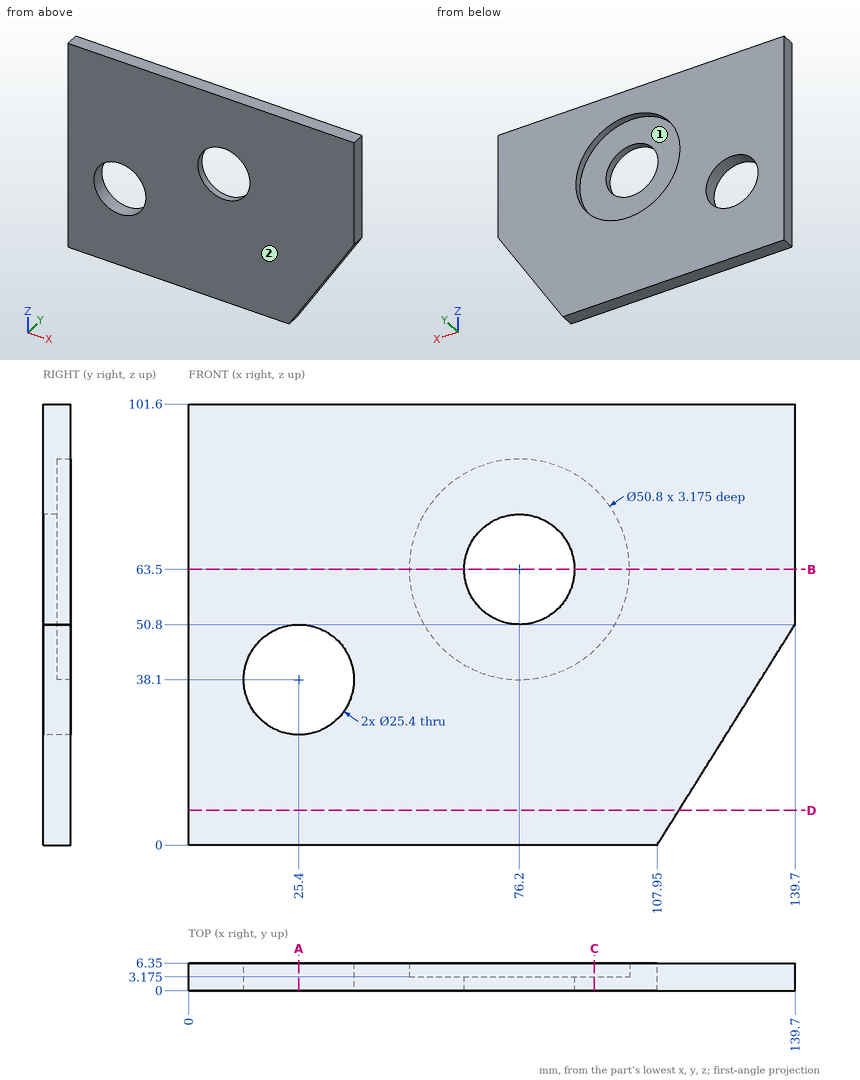
Check sheet for the drawn part. Datum: minimum x, y, z corner. Units: mm. Give positions to 0.01 mm unless a question says otherwise; leave off trailing zeros. Write each loop counter-clockwise with the first axis right and the second up, starting at its lowest first coordinate (ties: lowest second). Pieces come first, ordered by that corner, then holes. Notation, with made-up numbers: (42.5, -20.75) -> (62.5, -20.75) arc R14 ccw to (62.5, -5.75) -> close; hole circle Ø5 at (-39.75, 40.25). An arc over 180 degrees is marked (long way). Use one line per item in the form item = value. Start each with the question number.
1. Thickness scan on line 1 along X through (y, z) = (3.95, 63.5); line 2 along Z through (x, y) = (25.4, 2.75); line 3 along X through (y, z) = (3.5, 46). Record the ranges inside material, lowest first. Write a range as from..to.
2. Section check D-D (z = 8). Record the cut outline in (x, y), and give its area (3 significant figures).
3. Section check B-B (z = 63.5). Record the cut outline in (x, y) (3 decimals).
4. Section check A-A (x = 25.4). Record the cut outline in (y, z), and give its area (3 significant figures).
5. Mould release check, pull along Z, two halves, no side actions. Record for the marked faces 1 and 2: pulls with the +Z half, pulls with the -Z half, needs draft (parallel to the pull), parting line crosses it, or undercut.
6. Go/stop test with flat-tipped pins: P1, Ø15, axis at x = 76.2, z = 63.5, coming from the -Y side; P2, Ø1, axis at y = 1, z = 30, coming from the +X side; P3, Ø15, axis at x = 77.5, z = 75, coming from the +Y side (3 decimals). Record where each tip stops, or that it passes through.
7. Section check C-C (x = 93.5). Record the cut outline in (y, z) (3 decimals).
Conclusion:
q1.line_1 = 0..50.8, 101.6..139.7
q1.line_2 = 0..25.4, 50.8..101.6
q1.line_3 = 0..15.46, 35.34..57.79, 94.61..136.7
q2.outline = (0, 0) -> (112.95, 0) -> (112.95, 6.35) -> (0, 6.35) -> close
q2.area = 717 mm²
q3.outline = (0, 0) -> (63.5, 0) -> (63.5, 3.175) -> (50.8, 3.175) -> (50.8, 6.35) -> (0, 6.35) -> close; (88.9, 0) -> (139.7, 0) -> (139.7, 6.35) -> (101.6, 6.35) -> (101.6, 3.175) -> (88.9, 3.175) -> close
q4.outline = (0, 0) -> (6.35, 0) -> (6.35, 25.4) -> (0, 25.4) -> close; (0, 50.8) -> (6.35, 50.8) -> (6.35, 101.6) -> (0, 101.6) -> close
q4.area = 484 mm²
q5.face_1 = undercut
q5.face_2 = needs draft
q6.P1 = through
q6.P2 = 127.01
q6.P3 = 3.175
q7.outline = (0, 0) -> (6.35, 0) -> (6.35, 44.902) -> (3.175, 44.902) -> (3.175, 82.098) -> (6.35, 82.098) -> (6.35, 101.6) -> (0, 101.6) -> close
